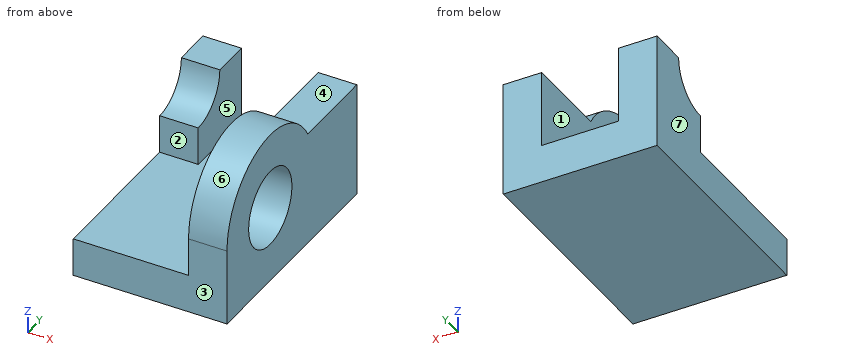
```python
from build123d import *

# Parameters (mm, degrees)
F0_W      = 1016
F0_H      = 254
F1_DEPTH  = 1524
F2_W      = 254
F2_H      = 508
F3_DEPTH  = 508
F4_W      = 254
F4_H      = 1524
F5_DEPTH  = 762
F7_DEPTH  = 254
F9_DEPTH  = 254
F10_W     = 508
F10_H     = 254
F11_DEPTH = 254


with BuildPart() as f1:
    # F0 (on Front) → F1 (new body)
    with BuildSketch(Plane.XZ):
        with Locations((332.7798564441, 16.3567224517)):
            Rectangle(F0_W, F0_H)
    extrude(amount=F1_DEPTH)

    # F2 (on face) → F3 (join)
    with BuildSketch(Plane.XY.offset(143.3567224517)):
        with Locations((-48.2201435559, -254)):
            Rectangle(F2_W, F2_H)
    extrude(amount=F3_DEPTH)

    # F4 (on face) → F5 (join)
    with BuildSketch(Plane.XY.offset(143.3567224517)):
        with Locations((713.7798564441, -762)):
            Rectangle(F4_W, F4_H)
    extrude(amount=F5_DEPTH)

    # F6 (on face) → F7 (cut)
    with BuildSketch(Plane(origin=(-175.2201435559, 0, 0), x_dir=(0, -1, 0), z_dir=(-1, 0, 0))):
        with BuildLine():
            Line((508, 651.3567224517), (254, 651.3567224517))
            ThreePointArc((254, 651.3567224517), (328.3948775786, 471.7516000304), (508, 397.3567224517))
            Line((508, 397.3567224517), (508, 651.3567224517))
        make_face()
    extrude(amount=-F7_DEPTH, mode=Mode.SUBTRACT)

    # F8 (on face) → F9 (cut)
    with BuildSketch(Plane.YZ.offset(840.7798564441)):
        with BuildLine():
            ThreePointArc((-1016, 651.3567224517), (-1195.6051224214, 576.9618448731), (-1270, 397.3567224517))
            Line((-1270, 397.3567224517), (-1016, 397.3567224517))
            Line((-1016, 397.3567224517), (-1016, 651.3567224517))
        make_face()
        with BuildLine():
            Line((-1016, 397.3567224517), (-762, 397.3567224517))
            ThreePointArc((-762, 397.3567224517), (-836.3948775786, 576.9618448731), (-1016, 651.3567224517))
            Line((-1016, 651.3567224517), (-1016, 397.3567224517))
        make_face()
        with BuildLine():
            Line((-1016, 397.3567224517), (-1270, 397.3567224517))
            ThreePointArc((-1270, 397.3567224517), (-1016, 143.3567224517), (-762, 397.3567224517))
            Line((-762, 397.3567224517), (-1016, 397.3567224517))
        make_face()
    extrude(amount=-F9_DEPTH, mode=Mode.SUBTRACT)

    # F10 (on face) → F11 (cut)
    with BuildSketch(Plane.YZ.offset(840.7798564441)):
        with BuildLine():
            Line((-762, 397.3567224517), (-1270, 397.3567224517))
            ThreePointArc((-1270, 397.3567224517), (-1016, 143.3567224517), (-762, 397.3567224517))
        make_face()
        with BuildLine():
            ThreePointArc((-762, 397.3567224517), (-1016, 651.3567224517), (-1270, 397.3567224517))
            Line((-1270, 397.3567224517), (-762, 397.3567224517))
        make_face()
        with BuildLine():
            Line((-1524, 905.3567224517), (-1524, 397.3567224517))
            ThreePointArc((-1524, 397.3567224517), (-1375.2102448427, 756.5669672945), (-1015.9999999999, 905.3567224517))
            Line((-1015.9999999999, 905.3567224517), (-1524, 905.3567224517))
        make_face()
        with BuildLine():
            Line((-508, 905.3567224517), (-1015.9999999999, 905.3567224517))
            ThreePointArc((-1015.9999999999, 905.3567224517), (-762, 837.2976275742), (-576.0590948775, 651.3567224517))
            Line((-576.0590948775, 651.3567224517), (-508, 651.3567224517))
            Line((-508, 651.3567224517), (-508, 905.3567224517))
        make_face()
        with Locations((-254, 778.3567224517)):
            Rectangle(F10_W, F10_H)
    extrude(amount=-F11_DEPTH, mode=Mode.SUBTRACT)


solid = f1.part
```
The listing builds one solid part. Answer for the finished solid, in the listing's coordinates (mm). Face numbers are marked on the shaded views. A direction names the side the tool comes from. Coordinates: 2 decimals unless noted, no trailing zeros. Loops run counter-clockwise (first coordinate to the right, second up) from the corner with the lowest first, then second, coordinate; pieces in that order, holes last. Notation, with made-up numbers: (83.25, 34) - (139.25, 34) arc R8 ccw to (139.25, 49) - close; hole circle Ø10 at (-26.5, 85.25). An arc over 180 degrees is marked (long way). Use a Markdown table: item, result. Add a question column.
1) The mould has two halves that part along X. Classify the marked faces 5, 6 and 7: released by +X, released by -X, zero draft, split by the parting line, or undercut.
2) Given pin 1 (10 mm diameter, centred on x = 655, y = -1063.5, fed in from +Z); pin 2 (10 mm diameter, centred on x = 199, y = -504, fed in from +Z), each flat-ended and moving along its own axis, determine where each tip first touches the part or whether it passes through.
3) The part is cut by section A-A, the plane y = -813. Give the vertices of the cut face in (x, z).
4) The part is cut by section C-C, the plane x = 767. Give the vertices of the cut face in (y, z).
5) Find the intervals of material crossed by line 1 (X direction, y = -433, z = 177); line 2 (Z direction, x = 694, y = -1016); line 3 (Z direction, x = 29.5, y = -521), in increasing order.
6) For the marked faces 1, 2, 3 and 4, determine the directions among +Z, -Z, +X, -X, +Y, -Y from which every point of the face is accessible in a straight line to the end or side of a thin tool.
7) The part is cut by section D-D, the plane x = 128.5. Give the vertices of the cut face in (y, z), and give its area (3 significant figures).
8) The part is cut by section B-B, the plane z = 505. Give the vertices of the cut face in (x, y), and give its area (3 significant figures).
Here are the results:
| question | item | result |
|---|---|---|
| 1 | face 5 | undercut |
| 1 | face 6 | zero draft |
| 1 | face 7 | released by -X |
| 2 | pin 1 | stops at z = 903.58 |
| 2 | pin 2 | stops at z = 143.36 |
| 3 | outline | (-175.22, -110.64) - (840.78, -110.64) - (840.78, 244.69) - (586.78, 244.69) - (586.78, 143.36) - (-175.22, 143.36) - close; (586.78, 550.02) - (840.78, 550.02) - (840.78, 863.03) - (586.78, 863.03) - close |
| 4 | outline | (-1524, -110.64) - (0, -110.64) - (0, 651.36) - (-576.06, 651.36) arc R508 ccw to (-1524, 397.36) - close; hole circle Ø508 at (-1016, 397.36) |
| 5 | line 1 | x = -175.22 to 78.78, 586.78 to 840.78 |
| 5 | line 2 | z = -110.64 to 143.36, 651.36 to 905.36 |
| 5 | line 3 | z = -110.64 to 143.36 |
| 6 | face 1 | +Z, +Y, -Y |
| 6 | face 2 | +Z, -X, -Y |
| 6 | face 3 | +Z, -Z, +X, -X, -Y |
| 6 | face 4 | +Z, +X, -X, +Y |
| 7 | outline | (-1524, -110.64) - (0, -110.64) - (0, 143.36) - (-1524, 143.36) - close |
| 7 | area | 387,000 mm^2 |
| 8 | outline | (-175.22, -300.4) - (78.78, -300.4) - (78.78, 0) - (-175.22, 0) - close; (586.78, -1512.46) - (840.78, -1512.46) - (840.78, -1246.06) - (586.78, -1246.06) - close; (586.78, -785.94) - (840.78, -785.94) - (840.78, 0) - (586.78, 0) - close |
| 8 | area | 344,000 mm^2 |
